```python
from build123d import *

# Parameters (mm, degrees)
F0_W      = 420
F0_H      = 420
F1_DEPTH  = 105
F2_T      = -6
F3_W      = 6
F3_H      = 408
F4_DEPTH  = 18
F5_W      = 6
F5_H      = 408
F6_DEPTH  = 18
F7_W      = 6
F7_H      = 18
F8_DEPTH  = 372
F9_W      = 6
F9_H      = 18
F10_DEPTH = 372
F11_W     = 408
F11_H     = 408
F11_W_2   = 400
F11_H_2   = 400
F12_DEPTH = 10
F14_W     = 400
F14_H     = 400
F15_DEPTH = 10
F16_DEPTH = 25.4


with BuildPart() as f1:
    # F0 (on Front) → F1 (new body, symmetric)
    with BuildSketch(Plane.XZ):
        Rectangle(F0_W, F0_H)
    extrude(amount=F1_DEPTH, both=True)

    # F2
    f2_openings = [f1.faces().sort_by_distance(p)[0] for p in [
        (0, -105, 0),
    ]]
    offset(amount=F2_T, openings=f2_openings)

    # F3 (on face) → F4 (join)
    with BuildSketch(Plane.YZ.offset(-204)):
        with Locations((-92, 0)):
            Rectangle(F3_W, F3_H)
    extrude(amount=F4_DEPTH)

    # F5 (on face) → F6 (join)
    with BuildSketch(Plane(origin=(204, 0, 0), x_dir=(0, -1, 0), z_dir=(-1, 0, 0))):
        with Locations((92, 0)):
            Rectangle(F5_W, F5_H)
    extrude(amount=F6_DEPTH)

    # F7 (on face) → F8 (join, through all)
    with BuildSketch(Plane.YZ.offset(-186)):
        with Locations((-92, 195)):
            Rectangle(F7_W, F7_H)
    extrude(amount=F8_DEPTH)

    # F9 (on face) → F10 (join, through all)
    with BuildSketch(Plane.YZ.offset(-186)):
        with Locations((-92, -195)):
            Rectangle(F9_W, F9_H)
    extrude(amount=F10_DEPTH)

    # F11 (on face) → F12 (join)
    with BuildSketch(Plane.XZ.offset(95)):
        Rectangle(F11_W, F11_H)
        Rectangle(F11_W_2, F11_H_2, mode=Mode.SUBTRACT)
    extrude(amount=F12_DEPTH)

    # F13: F1 across face


with BuildPart() as f1_1:
    add(f1.part)
    add(f1.part.mirror(Plane(origin=(0, 0, -210), x_dir=(1, 0, 0), z_dir=(0, 0, -1))))

    # F14 (on face) → F15 (join)
    with BuildSketch(Plane.XZ.offset(95)):
        with Locations((0, -420)):
            Rectangle(F14_W, F14_H)
    extrude(amount=F15_DEPTH)

    # F16 (cut): a face of the model
    f16_faces = [f1_1.faces().sort_by_distance(p)[0] for p in [
        (0, 5, -204),
    ]]
    extrude(f16_faces, amount=-F16_DEPTH, mode=Mode.SUBTRACT)


solid = f1_1.part
```
Build history of the part. All positions in model axes, mm. A direction names the side the tool comes from. Round coordinates to 2 decimals unless told otherwise and drop trailing zeros. Loops run counter-clockwise (first coordinate to the right, second up) from the corner with the lowest first, then second, coordinate; pieces in that order, holes last. Notation, with made-up numbers: M 1.25,19.25 L 21.25,19.25 A16 ccw 21.25,23.25 Z; hole C 48,-38 d6. An arc over 180 degrees is marked long. Answer as CSV lines item,"result".
1. Two-plate mould, pull along Z, no slides. Class faces 4 (the flat face through (-3, -1, 210)), 5 (the flat face through (210, -1, -204)), 6 (the flat face through (-3, 4, -624)): released by +Z, released by -Z, zero draft, split by the parting line, or undercut.
Resolved:
face 4,"released by +Z"
face 5,"zero draft"
face 6,"undercut"
2. Cut at B-B on x = 106.5. Write the cut outline in (y, z), then the cut area to 3 significant figures.
Resolved:
outline,"M -105,-630 L 105,-630 L 105,210 L -105,210 L -105,200 L -95,200 L -95,186 L -89,186 L -89,204 L 99,204 L 99,-624 L -89,-624 L -89,-606 L -95,-606 L -95,-234 L -89,-234 L -89,-186 L -95,-186 L -95,-200 L -105,-200 Z"
area,"12,300 mm²"
3. Wall check: probe 1 along Y at (x, z) = (10, -464); probe 2 along X at (y, z) = (74.5, 119); probe 3 along Z at (x, y) = (59.5, -60). Give the ranges that are in metal, low to high. Write a range as [from, to].
Resolved:
probe 1,"y = [-105, -95], [99, 105]"
probe 2,"x = [-210, -204], [204, 210]"
probe 3,"z = [-630, -624], [204, 210]"
4. Cut at A-A on y = 59.5. Write the cut outline in (x, z).
Resolved:
outline,"M -210,-630 L 210,-630 L 210,210 L -210,210 Z; hole M -204,-624 L 204,-624 L 204,204 L -204,204 Z"
5. 3-axis set-ups, long thin cutter, end or side, ignore diameter. For faces 1 (the flat face through (-3, -1, -630)), 2 (the flat face through (-3, -95, -417)), 3 (the flat face through (192, -95, -16)): which of +Z, -Z, +X, -X, +Y, -Y reach the whole face in a straight line?
Resolved:
face 1,"-Z, +X, -X, +Y, -Y"
face 2,"none"
face 3,"-Y"
6. Cut at C-C on z = -106.5. Write the cut outline in (x, y).
Resolved:
outline,"M -210,-105 L -200,-105 L -200,-95 L -186,-95 L -186,-89 L -204,-89 L -204,99 L 204,99 L 204,-89 L 186,-89 L 186,-95 L 200,-95 L 200,-105 L 210,-105 L 210,105 L -210,105 Z"
